from build123d import *

# Parameters (mm, degrees)
EXTRUDE_1_DEPTH             = 11
EXTRUDE_START               = -11
SKETCH_2_W                  = 74
SKETCH_2_H                  = 74
EXTRUDE_2_DEPTH             = 59
SKETCH_3_W                  = 48
SKETCH_3_H                  = 54
EXTRUDE_3_DEPTH             = 64
SKETCH_4_R                  = 27
EXTRUDE_4_DEPTH             = 5
FILLET_1_R                  = 10
SKETCH_7_R                  = 7.5
CUT_EXTRUDE_1_DEPTH         = 6
SKETCH_8_R                  = 4.5
CUT_EXTRUDE_2_DEPTH         = 128.910124697
SKETCH_9_R                  = 3
CUT_EXTRUDE_3_DEPTH         = 126.495019822
CUT_EXTRUDE_4_DEPTH         = 4
SKETCH_11_R                 = 37
EXTRUDE_5_DEPTH             = 3
CUT_EXTRUDE_START           = -45
SKETCH_14_W                 = 62
SKETCH_14_H                 = 62
CUT_EXTRUDE_6_DEPTH         = 35
SKETCH_13_R                 = 21
CUT_EXTRUDE_5_DEPTH         = 12
SKETCH_15_R                 = 23
SKETCH_15_R_2               = 21
EXTRUDE_6_DEPTH             = 12
CHAMFER_1_SIZE              = 2
CUT_EXTRUDE_7_REACH         = 133.488
SKETCH_12_R                 = 25
CUT_EXTRUDE_8_REACH         = 180.813
SKETCH_17_R                 = 15
CUT_EXTRUDE_9_DEPTH         = 2
M14X1_5_1_REACH             = 144.352
M14X1_5_1_BORE_R            = 6.25
HOLE_WIZARD_M6_1_D          = 5
HOLE_WIZARD_M6_1_DEPTH      = 10.497848452
HOLE_WIZARD_M6_1_TIP        = 1.502151548
SKETCH_25_R                 = 9
CUT_EXTRUDE_10_DEPTH        = 2
HOLE_START                  = 31
HOLE_WIZARD_M10_1_OUTLINE_R = 4.25
HOLE_WIZARD_M10_1_DEPTH     = 4
CUT_EXTRUDE_11_DEPTH        = 6


# Read off the part's stored shape, not the designer's step: M6 螺纹孔2, M10 螺纹孔1
with BuildPart() as part:
    # 草图1 → 凸台-拉伸1 (new body)
    with BuildSketch(Plane.XY):
        with BuildLine():
            Line((-91, -47), (45, -47))
            ThreePointArc((45, -47), (52.071067812, -44.071067812), (55, -37))
            Line((55, -37), (55, 37))
            ThreePointArc((55, 37), (52.071067812, 44.071067812), (45, 47))
            Line((45, 47), (-91, 47))
            ThreePointArc((-91, 47), (-98.071067812, 44.071067812), (-101, 37))
            Line((-101, 37), (-101, -37))
            ThreePointArc((-101, -37), (-98.071067812, -44.071067812), (-91, -47))
        make_face()
    extrude(amount=EXTRUDE_1_DEPTH)

    # 草图2 → 凸台-拉伸2 (add)
    with BuildSketch(Plane.XY.offset(11).offset(EXTRUDE_START)):
        Rectangle(SKETCH_2_W, SKETCH_2_H)
    extrude(amount=EXTRUDE_2_DEPTH)

    # 草图3 → 凸台-拉伸3 (add)
    with BuildSketch(Plane.ZY.offset(37)):
        with Locations((35, 0)):
            Rectangle(SKETCH_3_W, SKETCH_3_H)
    extrude(amount=EXTRUDE_3_DEPTH)

    # 草图4 → 凸台-拉伸4 (add)
    with BuildSketch(Plane.ZY.offset(101)):
        with Locations((32, 0)):
            Circle(SKETCH_4_R)
    extrude(amount=EXTRUDE_4_DEPTH)

    # 圆角1
    fillet_1_edges = [part.edges().sort_by_distance(p)[0] for p in [
        (-69, 27, 59),
        (-69, -27, 59),
    ]]
    fillet(fillet_1_edges, radius=FILLET_1_R)

    # 草图7 → 切除-拉伸1 (cut)
    with BuildSketch(Plane.XY.offset(11)):
        with Locations((45, 37)):
            Circle(SKETCH_7_R)
        with Locations((-75, 37)):
            Circle(SKETCH_7_R)
    cut_extrude_1 = extrude(amount=-CUT_EXTRUDE_1_DEPTH, mode=Mode.SUBTRACT)

    # 草图8 → 切除-拉伸2 (cut, through all)
    with BuildSketch(Plane.XY.offset(5)):
        with Locations((45, 37)):
            Circle(SKETCH_8_R)
        with Locations((-75, 37)):
            Circle(SKETCH_8_R)
    cut_extrude_2 = extrude(amount=-CUT_EXTRUDE_2_DEPTH, mode=Mode.SUBTRACT)

    # 镜向1: 切除-拉伸1, 切除-拉伸2 across plane
    add(cut_extrude_1.mirror(Plane.ZX), mode=Mode.SUBTRACT)
    add(cut_extrude_2.mirror(Plane.ZX), mode=Mode.SUBTRACT)

    # 草图9 → 切除-拉伸3 (cut, through all)
    with BuildSketch(Plane.XY.offset(11)):
        with Locations((45, 19)):
            Circle(SKETCH_9_R)
        with Locations((-57, -37)):
            Circle(SKETCH_9_R)
    extrude(amount=-CUT_EXTRUDE_3_DEPTH, mode=Mode.SUBTRACT)

    # 草图5 → 切除-拉伸4 (cut)
    with BuildSketch(Plane(origin=(0, 0, 0), x_dir=(-1, 0, 0), z_dir=(0, 0, -1))):
        with BuildLine():
            ThreePointArc((65, 37), (67.928932188, 29.928932188), (75, 27))
            Line((75, 27), (91, 27))
            Line((91, 27), (91, -27))
            Line((91, -27), (57, -27))
            ThreePointArc((57, -27), (49.928932188, -29.928932188), (47, -37))
            Line((47, -37), (-35, -37))
            ThreePointArc((-35, -37), (-37.928932188, -29.928932188), (-45, -27))
            Line((-45, -27), (-45, 9))
            ThreePointArc((-45, 9), (-37.928932188, 11.928932188), (-35, 19))
            Line((-35, 19), (-35, 37))
            Line((-35, 37), (65, 37))
        make_face()
    extrude(amount=-CUT_EXTRUDE_4_DEPTH, mode=Mode.SUBTRACT)

    # 草图11 → 凸台-拉伸5 (add)
    with BuildSketch(Plane.XY.offset(59)):
        Circle(SKETCH_11_R)
    extrude(amount=EXTRUDE_5_DEPTH)

    # 草图14 → 切除-拉伸6 (cut)
    with BuildSketch(Plane(origin=(0, 0, 4), x_dir=(-1, 0, 0), z_dir=(0, 0, -1)).offset(CUT_EXTRUDE_START)):
        Rectangle(SKETCH_14_W, SKETCH_14_H)
    extrude(amount=CUT_EXTRUDE_6_DEPTH, mode=Mode.SUBTRACT)

    # 草图13 → 切除-拉伸5 (cut)
    with BuildSketch(Plane(origin=(0, 0, 4), x_dir=(-1, 0, 0), z_dir=(0, 0, -1))):
        Circle(SKETCH_13_R)
    extrude(amount=-CUT_EXTRUDE_5_DEPTH, mode=Mode.SUBTRACT)

    # 草图15 → 凸台-拉伸6 (add)
    with BuildSketch(Plane(origin=(0, 0, 4), x_dir=(-1, 0, 0), z_dir=(0, 0, -1))):
        Circle(SKETCH_15_R)
        Circle(SKETCH_15_R_2, mode=Mode.SUBTRACT)
    extrude(amount=-EXTRUDE_6_DEPTH)

    # 倒角1
    chamfer_1_edges = [part.edges().sort_by_distance(p)[0] for p in [
        (21, 0, 16),
    ]]
    chamfer(chamfer_1_edges, length=CHAMFER_1_SIZE - 0.0001)  # a hair under: the kernel refuses the full size

    # 草图12 → 切除-拉伸7 (cut, up to next)
    with BuildSketch(Plane.XY.offset(62), mode=Mode.PRIVATE) as cut_extrude_7_sk1:
        Circle(SKETCH_12_R)
    cut_extrude_7_tool1 = extrude(cut_extrude_7_sk1.sketch, amount=-CUT_EXTRUDE_7_REACH, mode=Mode.PRIVATE) & part.part
    add(cut_extrude_7_tool1.solids().sort_by_distance((0, 0, 62))[0], mode=Mode.SUBTRACT)

    # 草图17 → 切除-拉伸8 (cut, up to next)
    with BuildSketch(Plane.ZY.offset(106), mode=Mode.PRIVATE) as cut_extrude_8_sk1:
        with Locations((32, 0)):
            Circle(SKETCH_17_R)
    cut_extrude_8_tool1 = extrude(cut_extrude_8_sk1.sketch, amount=-CUT_EXTRUDE_8_REACH, mode=Mode.PRIVATE) & part.part
    add(cut_extrude_8_tool1.solids().sort_by_distance((-106, 0, 32))[0], mode=Mode.SUBTRACT)

    # 草图18 → 切除-拉伸9 (cut)
    with BuildSketch(Plane.XZ.offset(27)):
        with BuildLine():
            Line((-101, 36.582575695), (-101, 32))
            Line((-101, 32), (-101, 27.417424305))
            ThreePointArc((-101, 27.417424305), (-80, 32), (-101, 36.582575695))
        make_face()
    cut_extrude_9 = extrude(amount=-CUT_EXTRUDE_9_DEPTH, mode=Mode.SUBTRACT)

    # M14x1.5 螺纹孔1 bore → M14x1.5 螺纹孔1 (cut, up to next)
    with BuildSketch(Plane.XZ.offset(25), mode=Mode.PRIVATE) as m14x1_5_1_sk1:
        with Locations((-91, 32)):
            Circle(M14X1_5_1_BORE_R)
    m14x1_5_1_tool1 = extrude(m14x1_5_1_sk1.sketch, amount=-M14X1_5_1_REACH, mode=Mode.PRIVATE) & part.part
    m14x1_5_1 = m14x1_5_1_tool1.solids().sort_by_distance((-91, -25, 32))[0]
    add(m14x1_5_1, mode=Mode.SUBTRACT)

    # 镜向2: 切除-拉伸9, M14x1.5 螺纹孔1 across plane
    add(cut_extrude_9.mirror(Plane.ZX), mode=Mode.SUBTRACT)
    add(m14x1_5_1.mirror(Plane.ZX), mode=Mode.SUBTRACT)

    # M6 螺纹孔1
    with Locations(Plane.XY.offset(62)):
        with Locations((30, 0), (0, -30), (-30, 0), (0, 30)):
            Hole(HOLE_WIZARD_M6_1_D / 2, depth=HOLE_WIZARD_M6_1_DEPTH)
            with Locations((0, 0, -(HOLE_WIZARD_M6_1_DEPTH + HOLE_WIZARD_M6_1_TIP / 2))):  # 118° drill point
                Cone(0, HOLE_WIZARD_M6_1_D / 2, HOLE_WIZARD_M6_1_TIP, mode=Mode.SUBTRACT)

    # M6 螺纹孔2 outline → M6 螺纹孔2 (revolve, cut)
    with BuildSketch(Plane(origin=(0, 17.320508076, 22), x_dir=(0, 1, 0), z_dir=(0, 0, -1))):
        Polygon((2.5, -92.502151548), (0, -91), (0, -106), (2.5, -106), align=None)
    revolve(axis=Axis((0, 17.320508076, 22), (1, 0, 0)), mode=Mode.SUBTRACT)

    # Hole Wizard M6 _2 2 outline → Hole Wizard M6 _2 2 (revolve, cut)
    with BuildSketch(Plane(origin=(0, -17.320508076, 22), x_dir=(0, 1, 0), z_dir=(0, 0, -1))):
        Polygon((2.5, -92.502151548), (0, -91), (0, -106), (2.5, -106), align=None)
    revolve(axis=Axis((0, -17.320508076, 22), (1, 0, 0)), mode=Mode.SUBTRACT)

    # Hole Wizard M6 _2 3 outline → Hole Wizard M6 _2 3 (revolve, cut)
    with BuildSketch(Plane.YX.offset(-52)):
        Polygon((2.5, -92.502151548), (0, -91), (0, -106), (2.5, -106), align=None)
    revolve(axis=Axis((0, 0, 52), (1, 0, 0)), mode=Mode.SUBTRACT)

    # 草图25 → 切除-拉伸10 (cut)
    with BuildSketch(Plane(origin=(0, 37, 0), x_dir=(1, 0, 0), z_dir=(0, 1, 0))):
        with Locations(Location((-24, -32, 0), (0, 0, 270))):
            Circle(SKETCH_25_R)
    extrude(amount=-CUT_EXTRUDE_10_DEPTH, mode=Mode.SUBTRACT)

    # M10 螺纹孔1 outline → M10 螺纹孔1 (cut)
    with BuildSketch(Plane(origin=(0, 0, 0), x_dir=(1, 0, 0), z_dir=(0, 1, 0)).offset(HOLE_START)):
        with Locations((-24, -32)):
            Circle(HOLE_WIZARD_M10_1_OUTLINE_R)
    extrude(amount=HOLE_WIZARD_M10_1_DEPTH, mode=Mode.SUBTRACT)

    # 草图16 → 切除-拉伸11 (cut)
    with BuildSketch(Plane(origin=(0, 0, 49), x_dir=(-1, 0, 0), z_dir=(0, 0, -1))):
        with BuildLine():
            Line((31, 31), (12, 31))
            Line((12, 31), (12, 27.49545417))
            ThreePointArc((12, 27.49545417), (21.213203436, 21.213203436), (27.49545417, 12))
            Line((27.49545417, 12), (31, 12))
            Line((31, 12), (31, 31))
        make_face()
        with BuildLine():
            Line((31, -31), (12, -31))
            Line((12, -31), (12, -27.49545417))
            ThreePointArc((12, -27.49545417), (21.213203436, -21.213203436), (27.49545417, -12))
            Line((27.49545417, -12), (31, -12))
            Line((31, -12), (31, -31))
        make_face()
        with BuildLine():
            Line((-31, 31), (-31, 12))
            Line((-31, 12), (-27.49545417, 12))
            ThreePointArc((-27.49545417, 12), (-21.213203436, 21.213203436), (-12, 27.49545417))
            Line((-12, 27.49545417), (-12, 31))
            Line((-12, 31), (-31, 31))
        make_face()
        with BuildLine():
            Line((-27.49545417, -12), (-31, -12))
            Line((-31, -12), (-31, -31))
            Line((-31, -31), (-12, -31))
            Line((-12, -31), (-12, -27.49545417))
            ThreePointArc((-12, -27.49545417), (-21.213203436, -21.213203436), (-27.49545417, -12))
        make_face()
    extrude(amount=-CUT_EXTRUDE_11_DEPTH, mode=Mode.SUBTRACT)


solid = part.part
Input: part model. Units: mm. Frame: model coordinates. A direction names the side the tool comes from. Coordinates: 2 decimals unless noted, no trailing zeros. Loops run counter-clockwise (first coordinate to the right, second up) from the corner with the lowest first, then second, coordinate; pieces in that order, holes last.
(1) Material intervals for probe 1 along Y at (x, z) = (-57, 6); probe 2 along X at (y, z) = (-4.5, 48.5); probe 3 along Y at (x, z) = (45, 9.7), sorted ascending.
(2) Pull-direction query (X, two-part tool) for faces 4 (the face through (28, -30, 59)), 5 (the face through (-101, 1, 4)), 6 (the face through (29, 12, 52)), 7 (the face through (37.85, -30.01, 1.97)); classes: released by +X, released by -X, zero draft, split by the parting line, or undercut.
(3) Section B-B on z = 32. Count the separate pieces of the cut face and the enclosed holes in it, then the cut area to 3 significant figures.
(4) Section A-A on x = -41.5. Return the cut outline in (y, z), then the cut area to 3 significant figures.
(5) First-contact query: pin 1 Ø11.5 at (x, y) = (-75, 37) entering from +Z; pin 2 Ø5 at (y, z) = (31, 33.5) entering from +X; pin 3 Ø5 at (x, y) = (-68, -23.5) entering from +Z. Flat tips, straight axial feed; report the tip coordinate or a pass-through.
(6) Set-up query: faces 1 (the face through (-12, 29, 52)), 2 (the face through (-95, 25, 27)), 3 (the face through (-99.16, -0.54, 49.56)). Return all of +Z, -Z, +X, -X, +Y, -Y with unobstructed straight access to the full face (end or side cutting, diameter ignored); none if empty.
Data:
1. probe 1: y = -47 to -40, -34 to 47
1. probe 2: x = -106 to -31, 31 to 37
1. probe 3: y = -47 to -44.5, -29.5 to 16, 22 to 29.5, 44.5 to 47
2. face 4: zero draft
2. face 5: released by -X
2. face 6: undercut
2. face 7: undercut
3. separate pieces: 4
3. enclosed holes: 0
3. area: 2,700 mm2
4. outline: (-47, 0) - (-37, 0) - (-37, 4) - (37, 4) - (37, 0) - (47, 0) - (47, 11) - (27, 11) - (27, 49) arc R10 ccw to (17, 59) - (-17, 59) arc R10 ccw to (-27, 49) - (-27, 11) - (-47, 11) - close; hole circle Ø30 at (0, 32)
4. area: 2,580 mm2
5. pin 1: stops at z = 5
5. pin 2: stops at x = 37
5. pin 3: stops at z = 58.17
6. face 1: none
6. face 2: +Y
6. face 3: -X
